```python
from build123d import *

# Parameters (mm, degrees)
CUT_EXTRUDE_1_DEPTH = 3


with BuildPart() as part:
    # Эскиз1 → Повернуть1 (revolve)
    with BuildSketch(Plane.XY):
        Polygon((3.5, 0), (1.8, 0), (1.8, 4), (1.5, 4.292679061), (1.5, 21.5), (3, 21.5), (3, 24), (3.75, 24), (3.75, 22.5), (5, 22.5), (5, 8.5), (4.5, 8.5), (4.5, 5), (4.6, 5), (4.6, 2), (3.5, 2), align=None)
    revolve(axis=Axis((0, 0, 0), (0, 1, 0)))

    # Эскиз3 → Вырез-Вытянуть1 (cut)
    with BuildSketch(Plane.XZ):
        with BuildLine():
            Line((0.046977339, 1.799386876), (0.31286893, 1.975376681))
            Line((0.31286893, 1.975376681), (0.51136302, 1.72583541))
            ThreePointArc((0.51136302, 1.72583541), (0.55623059, 1.711901729), (0.600719228, 1.696801818))
            Line((0.600719228, 1.696801818), (0.907980999, 1.782013048))
            Line((0.907980999, 1.782013048), (1.019647604, 1.483347149))
            ThreePointArc((1.019647604, 1.483347149), (1.058013454, 1.45623059), (1.095658534, 1.428121975))
            Line((1.095658534, 1.428121975), (1.414213562, 1.414213562))
            Line((1.414213562, 1.414213562), (1.428121975, 1.095658534))
            ThreePointArc((1.428121975, 1.095658534), (1.45623059, 1.058013454), (1.483347149, 1.019647604))
            Line((1.483347149, 1.019647604), (1.782013048, 0.907980999))
            Line((1.782013048, 0.907980999), (1.696801818, 0.600719228))
            ThreePointArc((1.696801818, 0.600719228), (1.711901729, 0.55623059), (1.72583541, 0.51136302))
            Line((1.72583541, 0.51136302), (1.975376681, 0.31286893))
            Line((1.975376681, 0.31286893), (1.799386876, 0.046977339))
            ThreePointArc((1.799386876, 0.046977339), (1.8, 0), (1.799386876, -0.046977339))
            Line((1.799386876, -0.046977339), (1.975376681, -0.31286893))
            Line((1.975376681, -0.31286893), (1.72583541, -0.51136302))
            ThreePointArc((1.72583541, -0.51136302), (1.711901729, -0.55623059), (1.696801818, -0.600719228))
            Line((1.696801818, -0.600719228), (1.782013048, -0.907980999))
            Line((1.782013048, -0.907980999), (1.483347149, -1.019647604))
            ThreePointArc((1.483347149, -1.019647604), (1.45623059, -1.058013454), (1.428121975, -1.095658534))
            Line((1.428121975, -1.095658534), (1.414213562, -1.414213562))
            Line((1.414213562, -1.414213562), (1.095658534, -1.428121975))
            ThreePointArc((1.095658534, -1.428121975), (1.058013454, -1.45623059), (1.019647604, -1.483347149))
            Line((1.019647604, -1.483347149), (0.907980999, -1.782013048))
            Line((0.907980999, -1.782013048), (0.600719228, -1.696801818))
            ThreePointArc((0.600719228, -1.696801818), (0.55623059, -1.711901729), (0.51136302, -1.72583541))
            Line((0.51136302, -1.72583541), (0.31286893, -1.975376681))
            Line((0.31286893, -1.975376681), (0.046977339, -1.799386876))
            ThreePointArc((0.046977339, -1.799386876), (0, -1.8), (-0.046977339, -1.799386876))
            Line((-0.046977339, -1.799386876), (-0.31286893, -1.975376681))
            Line((-0.31286893, -1.975376681), (-0.51136302, -1.72583541))
            ThreePointArc((-0.51136302, -1.72583541), (-0.55623059, -1.711901729), (-0.600719228, -1.696801818))
            Line((-0.600719228, -1.696801818), (-0.907980999, -1.782013048))
            Line((-0.907980999, -1.782013048), (-1.019647604, -1.483347149))
            ThreePointArc((-1.019647604, -1.483347149), (-1.058013454, -1.45623059), (-1.095658534, -1.428121975))
            Line((-1.095658534, -1.428121975), (-1.414213562, -1.414213562))
            Line((-1.414213562, -1.414213562), (-1.428121975, -1.095658534))
            ThreePointArc((-1.428121975, -1.095658534), (-1.45623059, -1.058013454), (-1.483347149, -1.019647604))
            Line((-1.483347149, -1.019647604), (-1.782013048, -0.907980999))
            Line((-1.782013048, -0.907980999), (-1.696801818, -0.600719228))
            ThreePointArc((-1.696801818, -0.600719228), (-1.711901729, -0.55623059), (-1.72583541, -0.51136302))
            Line((-1.72583541, -0.51136302), (-1.975376681, -0.31286893))
            Line((-1.975376681, -0.31286893), (-1.799386876, -0.046977339))
            ThreePointArc((-1.799386876, -0.046977339), (-1.8, 0), (-1.799386876, 0.046977339))
            Line((-1.799386876, 0.046977339), (-1.975376681, 0.31286893))
            Line((-1.975376681, 0.31286893), (-1.72583541, 0.51136302))
            ThreePointArc((-1.72583541, 0.51136302), (-1.711901729, 0.55623059), (-1.696801818, 0.600719228))
            Line((-1.696801818, 0.600719228), (-1.782013048, 0.907980999))
            Line((-1.782013048, 0.907980999), (-1.483347149, 1.019647604))
            ThreePointArc((-1.483347149, 1.019647604), (-1.45623059, 1.058013454), (-1.428121975, 1.095658534))
            Line((-1.428121975, 1.095658534), (-1.414213562, 1.414213562))
            Line((-1.414213562, 1.414213562), (-1.095658534, 1.428121975))
            ThreePointArc((-1.095658534, 1.428121975), (-1.058013454, 1.45623059), (-1.019647604, 1.483347149))
            Line((-1.019647604, 1.483347149), (-0.907980999, 1.782013048))
            Line((-0.907980999, 1.782013048), (-0.600719228, 1.696801818))
            ThreePointArc((-0.600719228, 1.696801818), (-0.55623059, 1.711901729), (-0.51136302, 1.72583541))
            Line((-0.51136302, 1.72583541), (-0.31286893, 1.975376681))
            Line((-0.31286893, 1.975376681), (-0.046977339, 1.799386876))
            ThreePointArc((-0.046977339, 1.799386876), (0, 1.8), (0.046977339, 1.799386876))
        make_face()
    extrude(amount=-CUT_EXTRUDE_1_DEPTH, mode=Mode.SUBTRACT)


solid = part.part
```
Source: CAD feature listing. Evaluate the final solid. Frame: model axes, mm. A direction names the side the tool comes from. Give positions to 0.01 mm unless a question says otherwise; leave off trailing zeros. Loops run counter-clockwise (first coordinate to the right, second up) from the corner with the lowest first, then second, coordinate; pieces in that order, holes last. Notation, with made-up numbers: (63, 2) -> (94, 2) arc R20 cw to (94, 39) -> close; hole circle Ø5 at (-23, 50.25). An arc over 180 degrees is marked (long way). Put each result on its own line as item: value. Start each with the question number.
1) Reachability of faces 4 (the face through (-2.41, 2, -2.75)), 5 (the face through (-3.746, 23.24, -0.165)), 6 (the face through (-1.5, 13.02, -0.07)) from +Z, -Z, +X, -X, +Y, -Y: full face, straight path, thin tool, end or side. Return the list, or none.
2) Cut plane C-C (x = 4). Return loops of the section in (y, z).
3) Contact query for flat-ended pins moving along their axis: P1, Ø3, axis at x = -2.5, z = -3.5, coming from the -Y side; P2, Ø3, axis at y = 2.5, z = -0.5, coming from the +X side; P3, Ø1, axis at y = 6.5, z = -1.5, coming from the -X side; P4, Ø1.5, axis at x = -0.5, z = -2, coming from the +Y side. Output: stop coordinate, or through.
4) Material intervals for probe 1 along X at (y, z) = (22.6, 0); probe 2 along X at (y, z) = (2.95, 0); probe 3 along Z at (x, y) = (0, 17), sorted ascending.
5) Cut plane D-D (z = 3.25). Return loops of the section in (x, y).
6) Cut plane B-B (z = 2.25). Return loops of the section in (x, y).
7) Cut plane A-A (y = 20). Return loops of the section in (x, z).
8) Draft query along Y for faces 1 (the face through (2, 0, 2)), 2 (the face through (-0.59, 6.73, -4.46)), 3 (the face through (-1.3, 21.5, 1.3)). Return one class per face: released by +Y, released by -Y, zero draft, split by the parting line, or undercut.
Results are:
1. face 4: -Y
1. face 5: +Y
1. face 6: +Y, -Y
2. outline: (2, -2.27) -> (5, -2.27) -> (5, -2.06) -> (8.5, -2.06) -> (8.5, -3) -> (22.5, -3) -> (22.5, 3) -> (8.5, 3) -> (8.5, 2.06) -> (5, 2.06) -> (5, 2.27) -> (2, 2.27) -> close
3. P1: stops at y = 0
3. P2: stops at x = 4.6
3. P3: stops at x = -4.39
3. P4: stops at y = 21.5
4. probe 1: x = -3.75 to -3, 3 to 3.75
4. probe 2: x = -4.6 to -1.8, 1.8 to 4.6
4. probe 3: z = -5 to -1.5, 1.5 to 5
5. outline: (-3.8, 8.5) -> (-3.11, 8.5) -> (-3.11, 5) -> (-3.26, 5) -> (-3.26, 2) -> (-1.3, 2) -> (-1.3, 0) -> (1.3, 0) -> (1.3, 2) -> (3.26, 2) -> (3.26, 5) -> (3.11, 5) -> (3.11, 8.5) -> (3.8, 8.5) -> (3.8, 22.5) -> (1.87, 22.5) -> (1.87, 24) -> (-1.87, 24) -> (-1.87, 22.5) -> (-3.8, 22.5) -> close
6. outline: (-4.47, 8.5) -> (-3.9, 8.5) -> (-3.9, 5) -> (-4.01, 5) -> (-4.01, 2) -> (-2.68, 2) -> (-2.68, 0) -> (2.68, 0) -> (2.68, 2) -> (4.01, 2) -> (4.01, 5) -> (3.9, 5) -> (3.9, 8.5) -> (4.47, 8.5) -> (4.47, 22.5) -> (3, 22.5) -> (3, 24) -> (1.98, 24) -> (1.98, 21.5) -> (-1.98, 21.5) -> (-1.98, 24) -> (-3, 24) -> (-3, 22.5) -> (-4.47, 22.5) -> close
7. outline: circle Ø10 at (0, 0); hole circle Ø3 at (0, 0)
8. face 1: released by -Y
8. face 2: undercut
8. face 3: released by +Y
